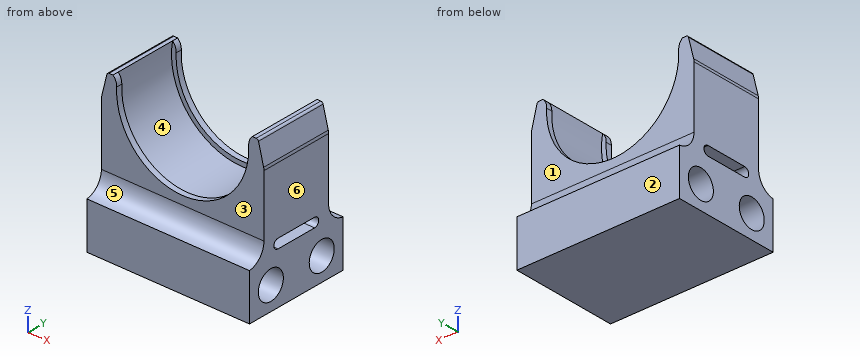
from build123d import *

# Parameters (mm, degrees)
BOSS_EXTRUDE2_DEPTH = 46
SKETCH4_R           = 6.15
CUT_EXTRUDE1_DEPTH  = 104.033974979
SKETCH6_W           = 45.215601595
SKETCH6_H           = 7.125
CUT_EXTRUDE2_DEPTH  = 104.033974979
CUT_EXTRUDE3_DEPTH  = 104.033974979
FILLET1_R           = 8
THICKEN1_START      = 7.125
THICKEN1_DEPTH      = 2.5
THICKEN2_START      = 36.375
THICKEN2_DEPTH      = 2.5
FILLET3_START       = 6
FILLET3_DEPTH       = 34
FILLET4_R           = 1


with BuildPart() as part:
    # Sketch3 → Boss-Extrude2 (new body)
    with BuildSketch(Plane(origin=(0, 0, 0), x_dir=(1, 0, 0), z_dir=(0, 1, 0))):
        with BuildLine():
            Line((35, 5.035917613), (35, 60))
            Line((35, 60), (-35, 60))
            Line((-35, 60), (-35, 5.035917613))
            Line((-35, 5.035917613), (-32.437862919, -5.215601595))
            Line((-32.437862919, -5.215601595), (-30, -5.215601595))
            ThreePointArc((-30, -5.215601595), (0, 30.45), (30, -5.215601595))
            Line((30, -5.215601595), (32.437862919, -5.215601595))
            Line((32.437862919, -5.215601595), (35, 5.035917613))
        make_face()
    extrude(amount=BOSS_EXTRUDE2_DEPTH)

    # Sketch4 → Cut-Extrude1 (cut, through all)
    with BuildSketch(Plane.ZY.offset(35)):
        with Locations((-50, 35.5)):
            Circle(SKETCH4_R)
        with Locations((-50, 10.5)):
            Circle(SKETCH4_R)
    extrude(amount=-CUT_EXTRUDE1_DEPTH, mode=Mode.SUBTRACT)

    # Sketch6 → Cut-Extrude2 (cut, through all)
    with BuildSketch(Plane.ZY.offset(35)):
        with Locations((-17.392199202, 42.4375)):
            Rectangle(SKETCH6_W, SKETCH6_H)
        with Locations((-17.392199202, 3.5625)):
            Rectangle(SKETCH6_W, SKETCH6_H)
    extrude(amount=-CUT_EXTRUDE2_DEPTH, mode=Mode.SUBTRACT)

    # Sketch7 → Cut-Extrude3 (cut, through all)
    with BuildSketch(Plane.ZY.offset(35)):
        with BuildLine():
            Line((-34, 32), (-34, 14))
            ThreePointArc((-34, 14), (-36, 12), (-38, 14))
            Line((-38, 14), (-38, 32))
            ThreePointArc((-38, 32), (-36, 34), (-34, 32))
        make_face()
    extrude(amount=-CUT_EXTRUDE3_DEPTH, mode=Mode.SUBTRACT)

    # Fillet1
    # the kernel refuses this fillet: 8 mm, written as the material it adds along each edge
    with BuildSketch(Plane(origin=(-35, 38.875, -40), x_dir=(0, 0, 1), z_dir=(1, 0, 0))) as fillet1_piece_1:
        with BuildLine():
            CenterArc((7.952004464, -8), FILLET1_R, 90, 83.720711677)
            Line((0, -7.125), (-0.159040089, -7.1075))
            ThreePointArc((-0.159040089, -7.1075), (-0.16, -3.5625), (-0.16, 0))
            Line((-0.16, 0), (0, 0.16))
            Line((0, 0.16), (7.952004464, 0.16))
            Line((7.952004464, 0.16), (7.952004464, 0))
        make_face()
    extrude(amount=70)
    with BuildSketch(Plane(origin=(-35, 7.125, -40), x_dir=(0, 0, 1), z_dir=(1, 0, 0))) as fillet1_piece_2:
        with BuildLine():
            CenterArc((7.952004464, 8), FILLET1_R, 186.279288323, 83.720711677)
            Line((0, 7.125), (-0.159040089, 7.1075))
            ThreePointArc((-0.159040089, 7.1075), (-0.16, 3.5625), (-0.16, 0))
            Line((-0.16, 0), (0, -0.16))
            Line((0, -0.16), (7.952004464, -0.16))
            Line((7.952004464, -0.16), (7.952004464, 0))
        make_face()
    extrude(amount=70)

    # Thicken1: read off the stored shape, not the designer's step
    # Thicken1 outline → Thicken1 (add)
    with BuildSketch(Plane(origin=(0, 0, 0), x_dir=(1, 0, 0), z_dir=(0, 1, 0)).offset(THICKEN1_START)):
        with BuildLine():
            Line((-30, -5.215601595), (-28.02955665, -4.873033346))
            add(Edge.make_bspline(
                [(-28.02955665, -4.873033346), (-28.098227513, -4.44491985), (-28.235569238, -3.588692857), (-28.415182418, -1.817508912), (-28.523288215, 1.384964463), (-27.97944925, 6.199907689), (-26.040449122, 12.009579762), (-22.790232653, 17.418782717), (-18.402164664, 21.998309903), (-11.490033606, 26.589068444), (-4.952214398, 28.293358132), (-0.733661392, 28.45), (0.733661392, 28.45), (4.952214398, 28.293358132), (11.490033606, 26.589068444), (18.402164664, 21.998309903), (22.790232653, 17.418782717), (26.040449122, 12.009579762), (27.97944925, 6.199907689), (28.523288215, 1.384964463), (28.415182418, -1.817508912), (28.235569238, -3.588692857), (28.098227513, -4.44491985), (28.02955665, -4.873033346)],
                knots=[0, 0, 0, 0, 0.01484375, 0.0296875, 0.059375, 0.11875, 0.178125, 0.2375, 0.296875, 0.35625, 0.475, 0.5, 0.5, 0.525, 0.64375, 0.703125, 0.7625, 0.821875, 0.88125, 0.940625, 0.9703125, 0.98515625, 1, 1, 1, 1], degree=3))
            Line((28.02955665, -4.873033346), (30, -5.215601595))
            ThreePointArc((30, -5.215601595), (0, 30.45), (-30, -5.215601595))
        make_face()
    extrude(amount=THICKEN1_DEPTH)

    # Thicken2: read off the stored shape, not the designer's step
    # Thicken2 outline → Thicken2 (add)
    with BuildSketch(Plane(origin=(0, 0, 0), x_dir=(1, 0, 0), z_dir=(0, 1, 0)).offset(THICKEN2_START)):
        with BuildLine():
            add(Edge.make_bspline(
                [(28.02955665, -4.873033346), (28.098227513, -4.44491985), (28.235569238, -3.588692857), (28.415182418, -1.817508912), (28.523288215, 1.384964463), (27.97944925, 6.199907689), (26.040449122, 12.009579762), (22.790232653, 17.418782717), (18.402164664, 21.998309903), (11.490033606, 26.589068444), (4.952214398, 28.293358132), (0.733661392, 28.45), (-0.733661392, 28.45), (-4.952214398, 28.293358132), (-11.490033606, 26.589068444), (-18.402164664, 21.998309903), (-22.790232653, 17.418782717), (-26.040449122, 12.009579762), (-27.97944925, 6.199907689), (-28.523288215, 1.384964463), (-28.415182418, -1.817508912), (-28.235569238, -3.588692857), (-28.098227513, -4.44491985), (-28.02955665, -4.873033346)],
                knots=[0, 0, 0, 0, 0.01484375, 0.0296875, 0.059375, 0.11875, 0.178125, 0.2375, 0.296875, 0.35625, 0.475, 0.5, 0.5, 0.525, 0.64375, 0.703125, 0.7625, 0.821875, 0.88125, 0.940625, 0.9703125, 0.98515625, 1, 1, 1, 1], degree=3))
            Line((28.02955665, -4.873033346), (30, -5.215601595))
            ThreePointArc((30, -5.215601595), (0, 30.45), (-30, -5.215601595))
            Line((-30, -5.215601595), (-28.02955665, -4.873033346))
        make_face()
    extrude(amount=THICKEN2_DEPTH)

    # Fillet3: read off the stored shape, not the designer's step
    # Fillet3 outline → Fillet3 (cut)
    with BuildSketch(Plane(origin=(0, 0, 0), x_dir=(1, 0, 0), z_dir=(0, 1, 0)).offset(FILLET3_START)):
        with BuildLine():
            Line((35, 5.035917613), (35, 5.651272685))
            ThreePointArc((35, 5.651272685), (34.962558609, 5.040525563), (34.850795181, 4.438925329))
            Line((34.850795181, 4.438925329), (35, 5.035917613))
        make_face()
        with BuildLine():
            Line((-35, 5.035917613), (-34.850795181, 4.438925329))
            ThreePointArc((-34.850795181, 4.438925329), (-34.962558609, 5.040525563), (-35, 5.651272685))
            Line((-35, 5.651272685), (-35, 5.035917613))
        make_face()
        with BuildLine():
            add(Edge.make_bspline(
                [(-28.02955665, -4.873033346), (-28.098227513, -4.44491985), (-28.235569238, -3.588692857), (-28.356138896, -2.399743128), (-28.403921261, -1.639675399), (-28.418446433, -1.328505626)],
                knots=[0, 0, 0, 0, 0.01484375, 0.0296875, 0.039856894, 0.039856894, 0.039856894, 0.039856894], degree=3))
            ThreePointArc((-28.418446433, -1.328505626), (-28.781681481, -3.446008708), (-30, -5.215601595))
            Line((-30, -5.215601595), (-28.02955665, -4.873033346))
        make_face()
        with BuildLine():
            ThreePointArc((30, -5.215601595), (28.781681481, -3.446008708), (28.418446433, -1.328505626))
            add(Edge.make_bspline(
                [(28.418446433, -1.328505626), (28.403921261, -1.639675399), (28.356138896, -2.399743128), (28.235569238, -3.588692857), (28.098227513, -4.44491985), (28.02955665, -4.873033346)],
                knots=[0.960143106, 0.960143106, 0.960143106, 0.960143106, 0.9703125, 0.98515625, 1, 1, 1, 1], degree=3))
            Line((28.02955665, -4.873033346), (30, -5.215601595))
        make_face()
    extrude(amount=FILLET3_DEPTH, mode=Mode.SUBTRACT)

    # Fillet4
    fillet4_edges = [part.edges().sort_by_distance(p)[0] for p in [
        (-32.437862919, 23, 5.215601595),
        (32.437862919, 23, 5.215601595),
    ]]
    fillet(fillet4_edges, radius=FILLET4_R)


solid = part.part
Work out the finished part from the listing and answer in its coordinate system (mm). Face numbers are marked on the shaded views. A direction names the side the tool comes from. Round coordinates to 2 decimals unless told otherwise and drop trailing zeros. Write each loop counter-clockwise with the first axis right and the second up, starting at its lowest first coordinate (ties: lowest second). Pieces come first, ordered by that corner, then holes.
1) Straight lines are drawn through the part: line 1 (Y direction, x = 19, z = -50); line 2 (Z direction, x = 25.5, y = 31); line 3 (Y direction, x = -21, z = -45.5). For each, find the intervals that lie inside material, in ascending order.
2) The mould has two halves that part along X. Classify the marked faces 4, 5 and 6: pulls with the +X half, pulls with the -X half, needs draft (parallel to the pull), parting line crosses it, or undercut.
3) A cutting plane is placed at B-B (z = -50). Give the vertices of the cut face in (x, y).
4) A cutting plane is placed at A-A (y = 23.5). Give the vertices of the cut face in (x, z).
5) Given pin 1 Ø7.5 at (y, z) = (35.5, -50) entering from +X; pin 2 Ø6 at (x, y) = (5, 40) entering from +Z; pin 3 Ø6 at (x, y) = (7.5, 27) entering from +Z; pin 4 Ø3 at (x, y) = (20.5, 33) entering from +Z, each flat-ended and moving along its own axis, determine where each tip first touches the part or whether it passes through.
6) A cutting plane is placed at C-C (z = -36). Give the vertices of the cut face in (x, y), plus the area to 3 significant figures.
7) A cutting plane is placed at D-D (y = 10.5). Give the vertices of the cut face in (x, z).
8) A tool of negligible diameter and unlimited length cuts with its end or side. For the marked faces 1, 2 and 3, from which of +Z, -Z, +X, -X, +Y, -Y can it reach the whole face along a straight path? Write none if from no direction.
Completed:
1. line 1: y = 0 to 4.35, 16.65 to 29.35, 41.65 to 46
1. line 2: z = -60 to -54.19, -45.81 to -38, -34 to -16.64
1. line 3: y = 0 to 6.31, 14.69 to 31.31, 39.69 to 46
2. face 4: undercut
2. face 5: needs draft
2. face 6: pulls with the +X half
3. outline: (-35, 0) - (35, 0) - (35, 4.35) - (-35, 4.35) - close; (-35, 16.65) - (35, 16.65) - (35, 29.35) - (-35, 29.35) - close; (-35, 41.65) - (35, 41.65) - (35, 46) - (-35, 46) - close
4. outline: (-35, -60) - (35, -60) - (35, -38) - (-35, -38) - close; (-35, -34) - (35, -34) - (35, -5.65) arc R5 ccw to (34.85, -4.44) - (32.63, 4.46) arc R1 ccw to (31.66, 5.22) - (30, 5.22) arc R30.45 cw (long way) to (-30, 5.22) - (-31.66, 5.22) arc R1 ccw to (-32.63, 4.46) - (-34.85, -4.44) arc R5 ccw to (-35, -5.65) - close
5. pin 1: passes through
5. pin 2: stops at z = -27.36
5. pin 3: stops at z = -28.58
5. pin 4: stops at z = -21.05
6. outline: (-35, 6.08) - (35, 6.08) - (35, 12) - (-35, 12) - close; (-35, 34) - (35, 34) - (35, 39.92) - (-35, 39.92) - close
6. area: 829 mm2
7. outline: (-35, -60) - (35, -60) - (35, -56.15) - (-35, -56.15) - close; (-35, -43.85) - (35, -43.85) - (35, -5.65) arc R5 ccw to (34.85, -4.44) - (32.63, 4.46) arc R1 ccw to (31.66, 5.22) - (30, 5.22) arc R30.45 cw (long way) to (-30, 5.22) - (-31.66, 5.22) arc R1 ccw to (-32.63, 4.46) - (-34.85, -4.44) arc R5 ccw to (-35, -5.65) - close
8. face 1: +Z, +X, -X, +Y
8. face 2: +Z, -Z, +X, -X, +Y
8. face 3: +Z, +X, -X, -Y
